Read the model definition and answer for the solid it produces. Units are mm, in the model's axes. Face numbers are marked on the shaded views. Coordinates: 2 decimals unless noted, no trailing zeros. Loops run counter-clockwise (first coordinate to the right, second up) from the corner with the lowest first, then second, coordinate; pieces in that order, holes last.
Q1. The mould has two halves that part along Z. Classify the marked faces 1, 2, 3 and 4: pulls with the +Z half, pulls with the -Z half, needs draft (parallel to the pull), parting line crosses it, or undercut.
Q2. Straight lines are drawn through the part: line 1 (X direction, y = -90.5, z = -74.5); line 2 (Y direction, x = -150, z = -75.5); line 3 (X direction, y = -9.5, z = 36). For each, find the intervals that lie inside material, in ascending order.
Q3. Section B-B (z = -95.5) is taken. Give the vertices of the cut face in (x, y).
Q4. Section C-C (x = -138) is taken. Give the vertices of the cut face in (y, z), then the cut area to 3 significant figures.
Q5. Section A-A (y = -33) is taken. Give the vertices of the cut face in (x, z).
Q6. Flat-ended cylindrical pins translate along their axes: P1, Ø3, axis at x = 2, z = -62, coming from the -Y side; P2, Ø3, axis at x = 2, z = -56, coming from the +Y side; P3, Ø5, axis at x = -67.5, z = -48.5, coming from the -Y side; P4, Ø3, axis at x = 1, y = -39.5, coming from the -Z side. Find the tip coordinate at first contact, or state that the pin passes through.
Q7. Section D-D (y = -118.5) is taken. Give the vertices of the cut face in (x, z).
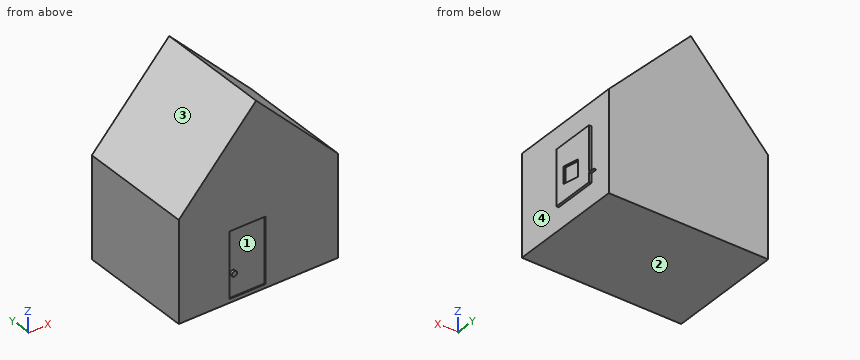
from build123d import *

# Parameters (mm, degrees)
F0_W     = 174.1194725037
F0_H     = 109.5531731844
F1_DEPTH = 127
F2_W     = 38.9005169272
F2_H     = 71.2012238801
F3_DEPTH = 1.27
F4_R     = 2.870090853
F5_DEPTH = 2.54
F7_DEPTH = 2.54


with BuildPart() as f1:
    # F0 (on Front) → F1 (new body)
    with BuildSketch(Plane.XZ):
        with Locations((-87.0597362518, -54.7765865922)):
            Rectangle(F0_W, F0_H)
        Polygon((-174.1194725037, 0), (0, 0), (-89.6153151989, 91.6864871979), align=None)
    extrude(amount=F1_DEPTH)

    # F2 (on face) → F3 (cut)
    with BuildSketch(Plane.XZ.offset(127)):
        with Locations((-98.9855192602, -69.9048843235)):
            Rectangle(F2_W, F2_H)
    extrude(amount=-F3_DEPTH, mode=Mode.SUBTRACT)

    # F4 (on face) → F5 (join)
    with BuildSketch(Plane.XZ.offset(125.73)):
        with Locations((-114.2556890845, -80.1247730851)):
            Circle(F4_R)
    extrude(amount=F5_DEPTH)

    # F6 (on face) → F7 (join)
    with BuildSketch(Plane.YZ):
        Polygon((-63.096486032, -25.4311673343), (-73.1122642756, -25.4311673343), (-73.1122642756, -47.0497577235), (-71.9686165237, -47.2507400464), (-63.096486032, -48.8099101597), align=None)
        Polygon((-41.3957126439, -25.4311673343), (-63.096486032, -25.4311673343), (-63.096486032, -48.8099101597), (-41.3957126439, -52.6235598049), align=None)
        Polygon((-71.9686165237, -47.2507400464), (-73.1122642756, -47.0497577235), (-73.1122642756, -65.521992743), (-63.096486032, -67.276372096), (-63.096486032, -48.8099101597), align=None)
        Polygon((-25.5374331027, -25.4311673343), (-41.3957126439, -25.4311673343), (-41.3957126439, -52.6235598049), (-25.5374331027, -55.4104615003), align=None)
        Polygon((-63.096486032, -67.276372096), (-73.1122642756, -65.521992743), (-73.1122642756, -85.3897556663), (-63.096486032, -85.3897556663), align=None)
        Polygon((-25.5374331027, -55.4104615003), (-41.3957126439, -52.6235598049), (-41.3957126439, -71.0775134402), (-25.5374331027, -73.8552744413), align=None)
        Polygon((-41.3957126439, -71.0775134402), (-63.096486032, -67.276372096), (-63.096486032, -85.3897556663), (-41.3957126439, -85.3897556663), align=None)
        Polygon((-25.5374331027, -73.8552744413), (-41.3957126439, -71.0775134402), (-41.3957126439, -85.3897556663), (-25.5374331027, -85.3897556663), (-25.5374331027, -75.1710534096), align=None)
        Polygon((-18.025631085, -75.1710534096), (-25.5374331027, -73.8552744413), (-25.5374331027, -75.1710534096), align=None)
    extrude(amount=F7_DEPTH)


solid = f1.part
Numbers:
1. face 1: undercut
1. face 2: pulls with the -Z half
1. face 3: pulls with the +Z half
1. face 4: needs draft
2. line 1: x = -174.12 to 0
2. line 2: y = -127 to 0
2. line 3: x = -140.94 to -35.19
3. outline: (-174.12, -127) - (-118.44, -127) - (-118.44, -125.73) - (-79.54, -125.73) - (-79.54, -127) - (0, -127) - (0, 0) - (-174.12, 0) - close
4. outline: (-127, -109.55) - (0, -109.55) - (0, 39.19) - (-127, 39.19) - close
4. area: 18,900 mm2
5. outline: (-174.12, -109.55) - (0, -109.55) - (0, -85.39) - (2.54, -85.39) - (2.54, -25.43) - (0, -25.43) - (0, 0) - (-89.62, 91.69) - (-174.12, 0) - close
6. P1: stops at y = -73.11
6. P2: stops at y = -25.54
6. P3: stops at y = -127
6. P4: stops at z = -109.55
7. outline: (-174.12, -109.55) - (0, -109.55) - (0, 0) - (-89.62, 91.69) - (-174.12, 0) - close
